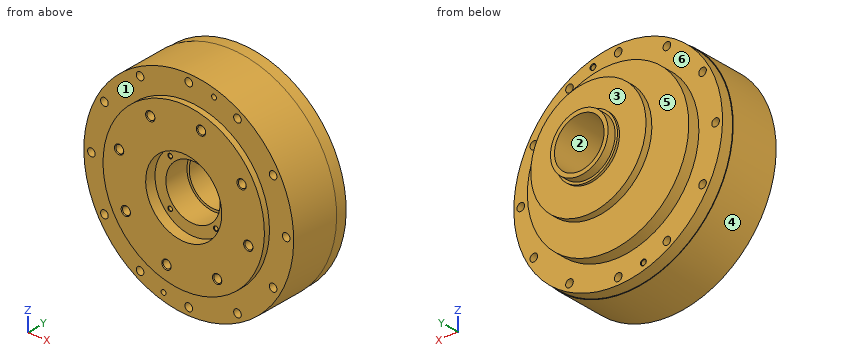
from build123d import *

# Parameters (mm, degrees)
SKETCH3_R                       = 3.3
CUT_EXTRUDE2_DEPTH              = 158.616623489
M8_TAPPED_HOLE1_D               = 6.8
M8_TAPPED_HOLE1_DEPTH           = 23.75
M8_TAPPED_HOLE1_CSINK_D         = 8.05
M8_TAPPED_HOLE1_CSINK_ANGLE     = 90
M8_TAPPED_HOLE1_TIP             = 2.042926105
M5X0_8_TAPPED_HOLE2_D           = 4.2
M5X0_8_TAPPED_HOLE2_CSINK_D     = 5.05
M5X0_8_TAPPED_HOLE2_CSINK_ANGLE = 90
M4_TAPPED_HOLE1_D               = 3.3
M4_TAPPED_HOLE1_DEPTH           = 20.1
M4_TAPPED_HOLE1_CSINK_D         = 4.05
M4_TAPPED_HOLE1_CSINK_ANGLE     = 90
M4_TAPPED_HOLE1_TIP             = 0.991420021


with BuildPart() as part:
    # Sketch1 → Revolve1 (revolve)
    with BuildSketch(Plane(origin=(0, 0, 0), x_dir=(0, 0, -1), z_dir=(1, 0, 0)), mode=Mode.PRIVATE) as revolve1_sk:
        Polygon((-33, 0), (-70, 0), (-70, 5), (-91, 5), (-91, 47.5), (-90.5, 47.5), (-90.5, 57.5), (-70, 57.5), (-70, 67.5), (-29.6, 67.5), (-29.6, 81.2), (-50, 81.2), (-50, 87), (-27, 87), (-27, 89), (-25, 89), (-25, 96), (-21.5, 96), (-21.5, 30), (-23.5, 30), (-23.5, 9.2), (-33, 9.2), align=None)
    revolve(revolve1_sk.sketch.rotate(Axis((0, -94.12, 0), (0, 1, 0)), 180), axis=Axis((0, -94.12, 0), (0, 1, 0)))

    # Sketch3 → Cut-Extrude2 (cut, through all)
    with BuildSketch(Plane.XZ.offset(-5)):
        with Locations(Location((-84.5, 0, 0), (0, 0, 270))):
            Circle(SKETCH3_R)
        with Locations(Location((-73.17914662, 42.25, 0), (0, 0, 270))):
            Circle(SKETCH3_R)
        with Locations(Location((-42.25, 73.17914662, 0), (0, 0, 270))):
            Circle(SKETCH3_R)
        with Locations(Location((0, 84.5, 0), (0, 0, 270))):
            Circle(SKETCH3_R)
        with Locations(Location((42.25, 73.17914662, 0), (0, 0, 270))):
            Circle(SKETCH3_R)
        with Locations(Location((73.17914662, 42.25, 0), (0, 0, 270))):
            Circle(SKETCH3_R)
        with Locations(Location((84.5, 0, 0), (0, 0, 270))):
            Circle(SKETCH3_R)
        with Locations(Location((73.17914662, -42.25, 0), (0, 0, 270))):
            Circle(SKETCH3_R)
        with Locations(Location((42.25, -73.17914662, 0), (0, 0, 270))):
            Circle(SKETCH3_R)
        with Locations(Location((0, -84.5, 0), (0, 0, 270))):
            Circle(SKETCH3_R)
        with Locations(Location((-42.25, -73.17914662, 0), (0, 0, 270))):
            Circle(SKETCH3_R)
        with Locations(Location((-73.17914662, -42.25, 0), (0, 0, 270))):
            Circle(SKETCH3_R)
    extrude(amount=-CUT_EXTRUDE2_DEPTH, mode=Mode.SUBTRACT)

    # M8 Tapped Hole1
    with Locations(Plane(origin=(0, 0, 0), x_dir=(-1, 0, 0), z_dir=(0, -1, 0))):
        with Locations((15.011504616, 56.023697925), (-29, 50.229473419), (-56.023697925, 15.011504616), (-50.229473419, -29), (-15.011504616, -56.023697925), (29, -50.229473419), (56.023697925, -15.011504616), (50.229473419, 29)):
            CounterSinkHole(M8_TAPPED_HOLE1_D / 2, M8_TAPPED_HOLE1_CSINK_D / 2, depth=M8_TAPPED_HOLE1_DEPTH, counter_sink_angle=M8_TAPPED_HOLE1_CSINK_ANGLE)
            with Locations((0, 0, -(M8_TAPPED_HOLE1_DEPTH + M8_TAPPED_HOLE1_TIP / 2))):  # 118° drill point
                Cone(0, M8_TAPPED_HOLE1_D / 2, M8_TAPPED_HOLE1_TIP, mode=Mode.SUBTRACT)

    # M5x0.8 Tapped Hole2 (through all)
    with Locations(Plane(origin=(0, 57.5, 0), x_dir=(1, 0, 0), z_dir=(0, 1, 0))):
        with Locations((-21.870209311, 81.620732321), (21.870209311, -81.620732321)):
            CounterSinkHole(M5X0_8_TAPPED_HOLE2_D / 2, M5X0_8_TAPPED_HOLE2_CSINK_D / 2, counter_sink_angle=M5X0_8_TAPPED_HOLE2_CSINK_ANGLE)

    # M4 Tapped Hole1
    with Locations(Plane(origin=(-19.798989873, 9.2, 19.798989873), x_dir=(0, 0, -1), z_dir=(0, -1, 0))):
        with Locations((0, 0), (0, 39.597979746), (39.597979746, 39.597979746), (39.597979746, 0)):
            CounterSinkHole(M4_TAPPED_HOLE1_D / 2, M4_TAPPED_HOLE1_CSINK_D / 2, depth=M4_TAPPED_HOLE1_DEPTH, counter_sink_angle=M4_TAPPED_HOLE1_CSINK_ANGLE)
            with Locations((0, 0, -(M4_TAPPED_HOLE1_DEPTH + M4_TAPPED_HOLE1_TIP / 2))):  # 118° drill point
                Cone(0, M4_TAPPED_HOLE1_D / 2, M4_TAPPED_HOLE1_TIP, mode=Mode.SUBTRACT)


solid = part.part
Work out the finished part from the listing and answer in its coordinate system (mm). Face numbers are marked on the shaded views. A direction names the side the tool comes from. Coordinates: 2 decimals unless noted, no trailing zeros. Write each loop counter-clockwise with the first axis right and the second up, starting at its lowest first coordinate (ties: lowest second). Pieces come first, ordered by that corner, then holes. Notation, with made-up numbers: M -32.5,-35.5 L -6.5,-35.5 A32 cw -6.5,-8.5 Z; hole C 75,-21.5 d9. An arc over 180 degrees is marked long. Use one line per item in the form item = value. Start each with the question number.
1. The part is cut by section A-A (y = 20). Give the number of separate pieces and of enclosed holes in the cut face, plus the area to 3 significant figures.
2. The part is cut by section C-C (x = -84.5). Give the vertices of the cut face in (y, z) (3 decimals).
3. Straight lines are drawn through the part: probe 1 along Y at (x, z) = (-9.5, -35.5); probe 2 along X at (y, z) = (46.5, 43); probe 3 along X at (y, z) = (45, -42). For each, find the intervals that lie inside material, in ascending order. Write a range as from..to.
4. The mould has two halves that part along Y. Classify the marked faces 4, 5 and 6: released by +Y, released by -Y, zero draft, split by the parting line, or undercut.
5. A tool of negligible diameter and unlimited length cuts with its end or side. For the marked faces 1, 2 and 3, from which of +Z, -Z, +X, -X, +Y, -Y can it reach the whole face along a straight path? Write none if from no direction.
6. The part is cut by section D-D (z = -42.25). Give the vertices of the cut face in (x, y).
7. Each of these flat-tipped pins is pushed along its axis until it touches: P1, Ø12, axis at y = 60, z = -49, coming from the -X side; P2, Ø7.5, axis at x = 73.18, z = -42.25, coming from the +Y side; P3, Ø2.5, axis at x = 19.8, z = 19.8, coming from the +Y side; P4, Ø11, axis at x = 56.02, z = -15.01, coming from the -Y side. Where does it stop, or does it pass through?
Evaluation:
q1.separate_pieces = 1
q1.enclosed_holes = 27
q1.area = 23,500 mm^2
q2.outline = M 5,-33.775 L 47.5,-33.775 L 47.5,-32.404 L 57.5,-32.404 L 57.5,-3.3 L 5,-3.3 Z; M 5,3.3 L 57.5,3.3 L 57.5,32.404 L 47.5,32.404 L 47.5,33.775 L 5,33.775 Z
q3.probe_1 = 0..67.5, 81.2..87
q3.probe_2 = -80.2..-76.39, -69.97..69.97, 76.39..80.2
q3.probe_3 = -80.73..-76.47, -69.89..69.89, 76.47..80.73
q4.face_4 = zero draft
q4.face_5 = undercut
q4.face_6 = released by +Y
q5.face_1 = -Y
q5.face_2 = +Y, -Y
q5.face_3 = +Y
q6.outline = M -80.6,5 L -76.48,5 L -76.48,57.5 L -80.03,57.5 L -80.03,47.5 L -80.6,47.5 Z; M -69.88,5 L -55.81,5 L -55.81,0 L 55.81,0 L 55.81,5 L 69.88,5 L 69.88,57.5 L 55.81,57.5 L 55.81,67.5 L -55.81,67.5 L -55.81,57.5 L -69.88,57.5 Z; M -26.74,81.2 L 26.74,81.2 L 26.74,87 L -26.74,87 Z; M 76.48,5 L 80.6,5 L 80.6,47.5 L 80.03,47.5 L 80.03,57.5 L 76.48,57.5 Z
q7.P1 = -79.33
q7.P2 = 57.5
q7.P3 = 89
q7.P4 = 0
